Here's how the part is built. I have some questions about the finished solid (model axes, mm). Coordinates: 2 decimals unless noted, no trailing zeros. Loops run counter-clockwise (first coordinate to the right, second up) from the corner with the lowest first, then second, coordinate; pieces in that order, holes last. Notation, with made-up numbers: M 78.5,22.25 L 89.5,22.25 A20 ccw 89.5,40.25 Z; hole C 69,27.25 d8. An arc over 180 degrees is marked long. Use one line per item in the form item = value. Start each with the question number.
(1) Imagine slicing it at B-B, the plane z = -14.4. Please give me the cut outline in (x, y).
(2) Will these pins go through, and if not, where does the flat tip stop? P1, Ø1.5, axis at x = 0.5, y = -34.5, coming from the -Z side; P2, Ø0.9, axis at x = -0.5, y = 34.5, coming from the +Z side; P3, Ø0.9, axis at x = -0.5, z = 52, coming from the +Y side.
(3) Imagine slicing it at C-C, the plane y = -4.5. Please give me the cut outline in (x, z).
(4) Please list where these lines run through material, in increasing order: L1, parallel to Y at x = 0.45, z = -4.6; L2, parallel to Y at x = 0.3, z = 16; L3, parallel to Z at x = -0.65, y = -13.
(5) Imagine slicing it at A-A, the plane y = -34. Please give me the cut outline in (x, z).
(6) Imagine slicing it at D-D, the plane x = -0.2. State how many separate pieces and enclosed holes the cut face has, and give its area (3 significant figures).
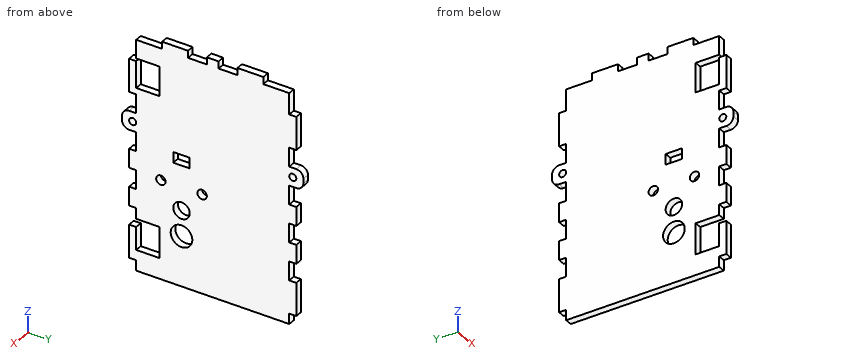
```python
from build123d import *

# Parameters (mm, degrees)
CROQUIS1_W               = 108
CROQUIS1_H               = 71
SALIENTE_EXTRUIR1_DEPTH  = 1.5
CROQUIS2_W               = 12
CROQUIS2_H               = 3
CROQUIS2_W_2             = 8
CORTAR_EXTRUIR1_DEPTH    = 3
CROQUIS4_W               = 8
CROQUIS4_H               = 3
SALIENTE_EXTRUIR2_DEPTH  = 3
REDONDEO1_R              = 3
CROQUIS5_R               = 1.5
CORTAR_EXTRUIR2_DEPTH    = 13
REDONDEO1_OF_SIMETR_A2_R = 3
CROQUIS6_W               = 3
CROQUIS6_H               = 14
CROQUIS6_H_2             = 8
CORTAR_EXTRUIR3_DEPTH    = 3
CROQUIS7_W               = 3.217414859
CROQUIS7_H               = 7.6
CORTAR_EXTRUIR4_DEPTH    = 73
CROQUIS8_R               = 1.5
CROQUIS8_R_2             = 2.5
CROQUIS8_R_3             = 3.6
CROQUIS8_W               = 2.5
CROQUIS8_H               = 6
CORTAR_EXTRUIR5_DEPTH    = 10
CROQUIS9_R               = 2
CROQUIS9_R_2             = 3.5
CROQUIS9_R_3             = 4.6
CROQUIS9_W               = 4.5
CROQUIS9_H               = 7
CORTAR_EXTRUIR6_DEPTH    = 10
CROQUIS10_W              = 13.122983438
CROQUIS10_H              = 10
CORTAR_EXTRUIR7_DEPTH    = 10
CROQUIS11_W              = 12.481361742
CROQUIS11_H              = 10
CORTAR_EXTRUIR8_DEPTH    = 10


with BuildPart() as part:
    # Croquis1 → Saliente-Extruir1 (new, symmetric)
    with BuildSketch(Plane(origin=(0, 0, 0), x_dir=(0, 0, -1), z_dir=(1, 0, 0))):
        Rectangle(CROQUIS1_W, CROQUIS1_H)
    extrude(amount=SALIENTE_EXTRUIR1_DEPTH, both=True)

    # Croquis2 → Cortar-Extruir1 (cut)
    with BuildSketch(Plane.ZY.offset(1.5)):
        with Locations((-48, -34)):
            Rectangle(CROQUIS2_W, CROQUIS2_H)
        with Locations((-24, -34)):
            Rectangle(CROQUIS2_W_2, CROQUIS2_H)
        with Locations((-8, -34)):
            Rectangle(CROQUIS2_W_2, CROQUIS2_H)
        with Locations((8, -34)):
            Rectangle(CROQUIS2_W_2, CROQUIS2_H)
        with Locations((24, -34)):
            Rectangle(CROQUIS2_W_2, CROQUIS2_H)
        with Locations((48, -34)):
            Rectangle(CROQUIS2_W, CROQUIS2_H)
        with Locations((48, 34)):
            Rectangle(CROQUIS2_W, CROQUIS2_H)
        with Locations((24, 34)):
            Rectangle(CROQUIS2_W_2, CROQUIS2_H)
        with Locations((8, 34)):
            Rectangle(CROQUIS2_W_2, CROQUIS2_H)
        with Locations((-8, 34)):
            Rectangle(CROQUIS2_W_2, CROQUIS2_H)
        with Locations((-24, 34)):
            Rectangle(CROQUIS2_W_2, CROQUIS2_H)
        with Locations((-48, 34)):
            Rectangle(CROQUIS2_W, CROQUIS2_H)
    extrude(amount=-CORTAR_EXTRUIR1_DEPTH, mode=Mode.SUBTRACT)

    # Croquis4 → Saliente-Extruir2 (add)
    with BuildSketch(Plane.ZY.offset(1.5)):
        with Locations((16, 37)):
            Rectangle(CROQUIS4_W, CROQUIS4_H)
    saliente_extruir2 = extrude(amount=-SALIENTE_EXTRUIR2_DEPTH)

    # Redondeo1
    redondeo1_edges = [part.edges().sort_by_distance(p)[0] for p in [
        (0, 38.5, 12),
        (0, 38.5, 20),
    ]]
    fillet(redondeo1_edges, radius=REDONDEO1_R)

    # Croquis5 → Cortar-Extruir2 (cut)
    with BuildSketch(Plane.ZY.offset(1.5)):
        with Locations((16, 34)):
            Circle(CROQUIS5_R)
    cortar_extruir2 = extrude(amount=-CORTAR_EXTRUIR2_DEPTH, mode=Mode.SUBTRACT)

    # Simetría2: Saliente-Extruir2, Cortar-Extruir2 across plane
    add(saliente_extruir2.mirror(Plane.ZX))
    add(cortar_extruir2.mirror(Plane.ZX), mode=Mode.SUBTRACT)

    # Redondeo1 of Simetría2
    redondeo1_of_simetr_a2_edges = [part.edges().sort_by_distance(p)[0] for p in [
        (0, -38.5, 12),
        (0, -38.5, 20),
    ]]
    fillet(redondeo1_of_simetr_a2_edges, radius=REDONDEO1_OF_SIMETR_A2_R)

    # Croquis6 → Cortar-Extruir3 (cut)
    with BuildSketch(Plane.ZY.offset(1.5)):
        with Locations((52.5, -28.5)):
            Rectangle(CROQUIS6_W, CROQUIS6_H)
        with Locations((52.5, -6.5)):
            Rectangle(CROQUIS6_W, CROQUIS6_H_2)
        with Locations((52.5, 6.5)):
            Rectangle(CROQUIS6_W, CROQUIS6_H_2)
        with Locations((52.5, 28.5)):
            Rectangle(CROQUIS6_W, CROQUIS6_H)
    extrude(amount=-CORTAR_EXTRUIR3_DEPTH, mode=Mode.SUBTRACT)

    # Croquis7 → Cortar-Extruir4 (cut)
    with BuildSketch(Plane(origin=(0, 32.5, 0), x_dir=(1, 0, 0), z_dir=(0, 1, 0))):
        with Locations((-0.10870743, 50.2)):
            Rectangle(CROQUIS7_W, CROQUIS7_H)
    extrude(amount=-CORTAR_EXTRUIR4_DEPTH, mode=Mode.SUBTRACT)

    # Croquis8 → Cortar-Extruir5 (cut)
    with BuildSketch(Plane(origin=(1.5, 0, 0), x_dir=(0, 0, -1), z_dir=(1, 0, 0))):
        with Locations((4.6, -4.5)):
            Circle(CROQUIS8_R)
        with Locations((4.6, -22)):
            Circle(CROQUIS8_R)
        with Locations((14.4, -13.25)):
            Circle(CROQUIS8_R_2)
        with Locations((25.2, -13.25)):
            Circle(CROQUIS8_R_3)
        with Locations((-6.85, -13.25)):
            Rectangle(CROQUIS8_W, CROQUIS8_H)
    extrude(amount=-CORTAR_EXTRUIR5_DEPTH, mode=Mode.SUBTRACT)

    # Croquis9 → Cortar-Extruir6 (cut)
    with BuildSketch(Plane.ZY.offset(1.5)):
        with Locations((-4.6, -22)):
            Circle(CROQUIS9_R)
        with Locations((-4.6, -4.5)):
            Circle(CROQUIS9_R)
        with Locations((-14.4, -13.25)):
            Circle(CROQUIS9_R_2)
        with Locations((-25.2, -13.25)):
            Circle(CROQUIS9_R_3)
        with Locations((6.85, -13.25)):
            Rectangle(CROQUIS9_W, CROQUIS9_H)
    extrude(amount=-CORTAR_EXTRUIR6_DEPTH, mode=Mode.SUBTRACT)

    # Croquis10 → Cortar-Extruir7 (cut)
    with BuildSketch(Plane.ZY.offset(1.5)):
        with Locations((-31.1, -27.5)):
            Rectangle(CROQUIS10_W, CROQUIS10_H)
    extrude(amount=-CORTAR_EXTRUIR7_DEPTH, mode=Mode.SUBTRACT)

    # Croquis11 → Cortar-Extruir8 (cut)
    with BuildSketch(Plane.ZY.offset(1.5)):
        with Locations((36.9, -27.5)):
            Rectangle(CROQUIS11_W, CROQUIS11_H)
    extrude(amount=-CORTAR_EXTRUIR8_DEPTH, mode=Mode.SUBTRACT)


solid = part.part
```
Answer:
q1.outline = M -1.5,-35.5 L 1.5,-35.5 L 1.5,-16.75 L -1.5,-16.75 Z; M -1.5,-9.75 L 1.5,-9.75 L 1.5,35.5 L -1.5,35.5 Z
q2.P1 = -42
q2.P2 = 42
q2.P3 = 21.5
q3.outline = M -1.5,-46.4 L 1.5,-46.4 L 1.5,-6.6 L -1.5,-6.6 Z; M -1.5,-2.6 L 1.5,-2.6 L 1.5,51 L -1.5,51 Z
q4.L1 = -32.5 to -24, -20 to -6.5, -2.5 to 32.5
q4.L2 = -38.5 to -35.5, -32.5 to 32.5, 35.5 to 38.5
q4.L3 = -46.4 to -29.79, -20.61 to -17.89, -10.91 to 4.6, 9.1 to 54
q5.outline = M -1.5,-42 L 1.5,-42 L 1.5,-28 L -1.5,-28 Z; M -1.5,-20 L 1.5,-20 L 1.5,-12 L -1.5,-12 Z; M -1.5,-4 L 1.5,-4 L 1.5,4 L -1.5,4 Z; M -1.5,12 L 1.5,12 L 1.5,14.5 L -1.5,14.5 Z; M -1.5,17.5 L 1.5,17.5 L 1.5,20 L -1.5,20 Z; M -1.5,28 L 1.5,28 L 1.5,42 L -1.5,42 Z
q6.separate_pieces = 1
q6.enclosed_holes = 7
q6.area = 6,330 mm²
